The model under review builds one solid part; all positions refer to its coordinate system, in mm. A direction names the side the tool comes from. Give positions to 0.01 mm unless a question says otherwise; leave off trailing zeros. Loops run counter-clockwise (first coordinate to the right, second up) from the corner with the lowest first, then second, coordinate; pieces in that order, holes last. Notation, with made-up numbers: M 70,-25 L 75,-25 A26 cw 75,1 Z; hole C -18.5,69.25 d7. An arc over 180 degrees is marked long. Write item = value, one per line. Start each with the question number.
1. We need section D-D on x = 48. Give the boundary of the cut face in (y, z).
2. Wall thickness on line 1 along X through (y, z) = (18.5, 1); line 2 along Y through (x, z) = (46, 0); line 3 along Y through (x, z) = (5, 5): over which ranges is each line inside the solid? List them lowest first. Write a range as from..to.
3. For pin 1 (4 mm diameter, centred on x = 52, y = 18, fed in from -Z); pin 2 (10 mm diameter, centred on x = 39, y = -13, fed in from -Z); pin 3 (3 mm diameter, centred on y = 18, z = 33.5, fed in from +X); pin 4 (23 mm diameter, centred on y = 0, z = 0, fed in from +X), all flat-tipped, find the tip position at first contact; note any pin that passes through.
4. We need section B-B on y = 11.5. Give the boundary of the cut face in (x, z) (3 decimals), then the cut area to 3 significant figures.
5. We need section A-A on y = 0. Give the boundary of the cut face in (x, z).
6. We need section C-C on z = 6.5. Give the boundary of the cut face in (x, y) (3 decimals).
7. Draft analysis for pull direction X (two halves, no side actions). For faces 4 (the face through (70, -16, 9.525)), 5 (the face through (76.2, 5, -12)), 6 (the face through (57, 16, -9.525)), state which applies: pulls with the +X half, pulls with the -X half, needs draft (parallel to the pull), parting line crosses it, or undercut.
8. For faces 1 (the face through (6, -12.7, 30)), 2 (the face through (70, 16, 9.525)), 3 (the face through (63.5, -19, 0)), list the 3-axis set-ups (+Z, -Z, +X, -X, +Y, -Y) from which the entire face can be reached by the end or side of a thin tool; tool diameter is ignored.
from build123d import *
from build123d import SkipClean  # not in build123d's __all__

# Parameters (mm, degrees)
F0_R          = 25.4
F0_R_2        = 12.7
F1_DEPTH      = 76.2
F3_DEPTH      = 25.4
F5_DEPTH      = 12.7
F5_DEPTH_BACK = 25.4
F6_R          = 12.7
F7_DEPTH      = 38.1


with BuildPart() as f1:
    # F0 (on Right) → F1 (new body)
    with BuildSketch(Plane.YZ):
        Circle(F0_R)
        Circle(F0_R_2, mode=Mode.SUBTRACT)
    extrude(amount=F1_DEPTH)

    # F2 (on Front) → F3 (cut, symmetric)
    with BuildSketch(Plane.XZ):
        Polygon((76.2, 9.525), (76.2, 25.4), (50.8, 25.4), (50.8, -9.525), (63.5, -9.525), (63.5, 9.525), align=None)
    extrude(amount=F3_DEPTH, both=True, mode=Mode.SUBTRACT)

    # F4 (on Front) → F5 (join, two sides)
    with BuildSketch(Plane.XZ) as f5_sk:
        Polygon((0, 50.8), (0, 0), (38.1, 0), align=None)
    extrude(amount=F5_DEPTH)
    extrude(f5_sk.sketch, amount=-F5_DEPTH_BACK)

    # F6 (on Right) → F7 (cut)
    with BuildSketch(Plane.YZ):
        Circle(F6_R)
    with SkipClean():  # cleaning this boolean's faces spoils the solid; the shape is the same uncleaned
        extrude(amount=F7_DEPTH, mode=Mode.SUBTRACT)


solid = f1.part
Final values:
q1.outline = C 0,0 d50.8; hole C 0,0 d25.4
q2.line_1 = 0..50.8, 63.5..76.2
q2.line_2 = -25.4..-12.7, 12.7..25.4
q2.line_3 = -24.9..-11.67, 11.67..25.4
q3.pin_1 = -19.73
q3.pin_2 = -24.11
q3.pin_3 = 14.1
q3.pin_4 = through
q4.outline = M 0,-22.648 L 76.2,-22.648 L 76.2,-5.389 L 63.5,-5.389 L 63.5,-9.525 L 50.8,-9.525 L 50.8,-5.389 L 0,-5.389 Z; M 0,5.389 L 50.8,5.389 L 50.8,22.648 L 21.114,22.648 L 0,50.8 Z; M 63.5,5.389 L 76.2,5.389 L 76.2,9.525 L 63.5,9.525 Z
q4.area = 2,490 mm²
q5.outline = M 0,-25.4 L 76.2,-25.4 L 76.2,-12.7 L 0,-12.7 Z; M 0,12.7 L 50.8,12.7 L 50.8,25.4 L 19.05,25.4 L 0,50.8 Z
q6.outline = M 0,-24.554 L 50.8,-24.554 L 50.8,-10.911 L 0,-10.911 Z; M 0,10.911 L 50.8,10.911 L 50.8,24.554 L 33.225,24.554 L 33.225,25.4 L 0,25.4 Z; M 63.5,-24.554 L 76.2,-24.554 L 76.2,-10.911 L 63.5,-10.911 Z; M 63.5,10.911 L 76.2,10.911 L 76.2,24.554 L 63.5,24.554 Z
q7.face_4 = needs draft
q7.face_5 = pulls with the +X half
q7.face_6 = undercut
q8.face_1 = +Z, +X, -X, -Y
q8.face_2 = +Z, +X, +Y, -Y
q8.face_3 = +Z, +Y, -Y
